The listing builds one solid part. Answer for the finished solid, in the listing's coordinates (mm). A direction names the side the tool comes from. Give positions to 0.01 mm unless a question says otherwise; leave off trailing zeros. Loops run counter-clockwise (first coordinate to the right, second up) from the corner with the lowest first, then second, coordinate; pieces in that order, holes last. Notation, with made-up numbers: (-11.75, -9) - (25.25, -9) arc R37 cw to (25.25, 27) - close; hole circle Ø9 at (-3.75, 21.5). An arc over 180 degrees is marked (long way). Write item = value, one per line. Start each with the question number.
1) The part is cut by section A-A on x = -44.45. Write down the section's boundary in (y, z) (3 decimals), plus the area to 3 significant figures.
2) The part is cut by section D-D on x = -5. State how many separate pieces and enclosed holes the cut face has, plus the area to 3 significant figures.
3) The part is cut by section B-B on z = 11. Write down the section's boundary in (x, y), plus the area to 3 significant figures.
4) Flat-ended cylindrical pins translate along their axes: P1, Ø17.5, axis at x = -1.5, z = -1, coming from the -Y side; P2, Ø12, axis at y = 27, z = 2, coming from the +X side; P3, Ø14.5, axis at x = -44.45, y = 6.35, coming from the +Z side; P4, Ø10, axis at y = -6.5, z = -3.5, coming from the +X side. Find the tip coordinate at first contact, or state that the pin passes through.
5) Which of the six approach directions +Z, -Z, +X, -X, +Y, -Y give full straight-line access (tool end or side, diameter ignored) to faces 4 (the flat face through (-6, 17.526, 0)), 5 (the cylindrical face through (-5.05, -3.88, -12.02))?
6) The mould has two halves that part along Z. Classify faces 1 (the cylindrical face through (-40.18, 13.05, -0.22)), 2 (the cylindrical face through (-25.59, 2.2, -0.18)), 3 (the flat face through (-68, 10, -15.875)): +Z half, -Z half, draft (parallel to the pull), parting line (faces both ways), or undercut.
7) The part is cut by section C-C on z = 0. Write down the section's boundary in (x, y), plus the area to 3 significant figures.
8) Consider probe 1 along Y at (x, z) = (0, -10.5); probe 2 along Z at (x, y) = (-18, 0.5) (3 decimals); probe 3 along X at (y, z) = (0, 12). Determine where each line is inside the solid, lowest interval first.
from build123d import *

# Parameters (mm, degrees)
SKETCH11_W         = 158.75
SKETCH11_H         = 44.45
SKETCH11_R         = 6.36905
SKETCH11_R_2       = 7.94385
EXTRUDE3_DEPTH     = 15.875
CUT_EXTRUDE1_DEPTH = 30.226
FILLET1_R          = 12.7


with BuildPart() as part:
    # Sketch11 → Extrude3 (new body, symmetric)
    with BuildSketch(Plane.XY):
        with Locations((-66.675, 9.525)):
            Rectangle(SKETCH11_W, SKETCH11_H)
        Circle(SKETCH11_R, mode=Mode.SUBTRACT)
        with Locations((-44.45, 6.35)):
            Circle(SKETCH11_R_2, mode=Mode.SUBTRACT)
    extrude(amount=EXTRUDE3_DEPTH, both=True)

    # Sketch12 → Cut-Extrude1 (cut)
    with BuildSketch(Plane.XZ.offset(12.7)):
        with BuildLine():
            Line((-17.526, 8.0645), (12.7, 8.0645))
            Line((12.7, 8.0645), (12.7, -8.0645))
            Line((12.7, -8.0645), (-17.526, -8.0645))
            ThreePointArc((-17.526, -8.0645), (-25.5905, 0), (-17.526, 8.0645))
        make_face()
    extrude(amount=-CUT_EXTRUDE1_DEPTH, mode=Mode.SUBTRACT)

    # Fillet1
    fillet1_edges = [part.edges().sort_by_distance(p)[0] for p in [
        (12.7, -12.7, -11.96975),
        (12.7, 31.75, 0),
        (12.7, -12.7, 11.96975),
    ]]
    fillet(fillet1_edges, radius=FILLET1_R)


solid = part.part
Answer below:
q1.outline = (-12.7, -15.875) - (-1.594, -15.875) - (-1.594, 15.875) - (-12.7, 15.875) - close; (14.294, -15.875) - (31.75, -15.875) - (31.75, 15.875) - (14.294, 15.875) - close
q1.area = 907 mm2
q2.separate_pieces = 3
q2.enclosed_holes = 0
q2.area = 801 mm2
q3.outline = (-146.05, -12.7) - (0, -12.7) arc R12.7 ccw to (12.7, 0) - (12.7, 19.05) arc R12.7 ccw to (0, 31.75) - (-146.05, 31.75) - close; hole circle Ø15.89 at (-44.45, 6.35); hole circle Ø12.74 at (0, 0)
q3.area = 6,660 mm2
q4.P1 = -12.7
q4.P2 = 12.55
q4.P3 = through
q4.P4 = 11.89
q5.face_4 = +X, -Y
q5.face_5 = +Z, -Z
q6.face_1 = draft
q6.face_2 = undercut
q6.face_3 = -Z half
q7.outline = (-146.05, -12.7) - (-25.59, -12.7) - (-25.59, 17.53) - (12.7, 17.53) - (12.7, 19.05) arc R12.7 ccw to (0, 31.75) - (-146.05, 31.75) - close; hole circle Ø15.89 at (-44.45, 6.35)
q7.area = 5,670 mm2
q8.probe_1 = -12.7 to -6.37, 6.37 to 31.75
q8.probe_2 = -15.875 to -8.051, 8.051 to 15.875
q8.probe_3 = -146.05 to -49.22, -39.68 to -6.37, 6.37 to 12.7
